Can you work these out from the model? Positions are in its coordinate system, mm. Coordinates: 2 decimals unless noted, no trailing zeros. Order: outer loops, then holes, each group sorted by start corner. A loop starts at its lowest first (then second) coordinate and runs counter-clockwise, first axis right, second up. Notation, with made-up numbers: (-10, 64) -> (23, 64) arc R4 cw to (23, 69) -> close; hole circle Ø6 at (85.25, 14.5). An arc over 180 degrees is marked (long way). Answer as a JSON object with one key per item and string values. Group by question number.
(1) I need wall thicknesses on line 1 (X direction, y = 1.25, z = -0.25); line 2 (X direction, y = 2.05, z = 0.25); line 3 (X direction, y = 1.55, z = 1.5). Which ranges of each line are inside material? Lowest first, please.
(2) I want a section at D-D, the plane x = 15.5. List the corners of the cut face in (y, z) for me, plus the area to 3 significant figures.
(3) I want a section at C-C, the plane z = 0.5. List the corners of the cut face in (x, y) for me, plus the area to 3 significant figures.
(4) For pin 1 (1.9 mm diameter, centred on x = -25, z = -0.25, fed in from +Y) (3 decimals), with a flat end and sliding along its axis, tell me the tip position at first contact or that it passes through.
(5) I want a section at B-B, the plane y = 1.1. List the corners of the cut face in (x, z) for me.
(6) I want a section at A-A, the plane x = 25. List the corners of the cut face in (y, z) for me.
from build123d import *

# Parameters (mm, degrees)
SKETCH_1_W          = 60
SKETCH_1_H          = 9.5
EXTRUDE_1_DEPTH     = 3
SKETCH_2_R          = 1.6
CUT_EXTRUDE_1_DEPTH = 3
FILLET_1_R          = 2


with BuildPart() as part:
    # 草图1 → 凸台-拉伸1 (new body)
    with BuildSketch(Plane(origin=(0, 0, 0), x_dir=(1, 0, 0), z_dir=(0, 1, 0))):
        Rectangle(SKETCH_1_W, SKETCH_1_H)
    extrude(amount=EXTRUDE_1_DEPTH)

    # 草图2 → 切除-拉伸1 (cut)
    with BuildSketch(Plane(origin=(0, 3, 0), x_dir=(1, 0, 0), z_dir=(0, 1, 0))):
        with Locations(Location((-16.5, -0.25, 0), (0, 0, 270))):
            Circle(SKETCH_2_R)
        with Locations(Location((-25, 0.25, 0), (0, 0, 270))):
            Circle(SKETCH_2_R)
        with Locations(Location((25, 0.25, 0), (0, 0, 90))):
            Circle(SKETCH_2_R)
        with Locations(Location((16.5, -0.25, 0), (0, 0, 90))):
            Circle(SKETCH_2_R)
    extrude(amount=-CUT_EXTRUDE_1_DEPTH, mode=Mode.SUBTRACT)

    # 圆角1
    fillet_1_edges = [part.edges().sort_by_distance(p)[0] for p in [
        (-30, 1.5, -4.75),
        (30, 1.5, -4.75),
        (30, 1.5, 4.75),
        (-30, 1.5, 4.75),
    ]]
    fillet(fillet_1_edges, radius=FILLET_1_R)


solid = part.part
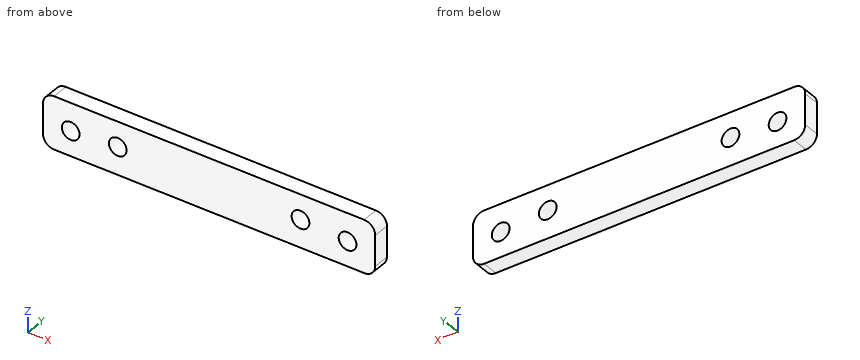
Computed values:
{
 "1": {"line 1": "x = -30 to -26.6, -23.4 to -18.02, -14.98 to 14.98, 18.02 to 23.4, 26.6 to 30", "line 2": "x = -30 to -26.52, -23.48 to -18.1, -14.9 to 14.9, 18.1 to 23.48, 26.52 to 30", "line 3": "x = -30 to -17.5, -15.5 to 15.5, 17.5 to 30"},
 "2": {"outline": "(0, -4.75) -> (3, -4.75) -> (3, -1) -> (0, -1) -> close; (0, 1.5) -> (3, 1.5) -> (3, 4.75) -> (0, 4.75) -> close", "area": "21.0 mm2"},
 "3": {"outline": "(-30, 0) -> (-26.41, 0) -> (-26.41, 3) -> (-30, 3) -> close; (-23.59, 0) -> (-18.08, 0) -> (-18.08, 3) -> (-23.59, 3) -> close; (-14.92, 0) -> (14.92, 0) -> (14.92, 3) -> (-14.92, 3) -> close; (18.08, 0) -> (23.59, 0) -> (23.59, 3) -> (18.08, 3) -> close; (26.41, 0) -> (30, 0) -> (30, 3) -> (26.41, 3) -> close", "area": "144 mm2"},
 "4": {"pin 1": "passes through"},
 "5": {"outline": "(-30, -2.75) arc R2 ccw to (-28, -4.75) -> (28, -4.75) arc R2 ccw to (30, -2.75) -> (30, 2.75) arc R2 ccw to (28, 4.75) -> (-28, 4.75) arc R2 ccw to (-30, 2.75) -> close; hole circle Ø3.2 at (-25, -0.25); hole circle Ø3.2 at (-16.5, 0.25); hole circle Ø3.2 at (16.5, 0.25); hole circle Ø3.2 at (25, -0.25)"},
 "6": {"outline": "(0, -4.75) -> (3, -4.75) -> (3, -1.85) -> (0, -1.85) -> close; (0, 1.35) -> (3, 1.35) -> (3, 4.75) -> (0, 4.75) -> close"}
}
